Could you check a few things on this drawing? It's one solid part, dimensions in mm from its lowest x, y, z. A direction names the side the tool comes from. Give positions to 0.01 mm unless a question says otherwise; leave off trailing zeros. Loops run counter-clockwise (first coordinate to the right, second up) from the corner with the lowest first, then second, coordinate; pieces in that order, holes last.
1. Imagine slicing it at D-D (z = 23). List the corners of the cut face in (x, y) for me.
2. For the marked faces 1 and 2, which set-ups out of +Z, -Z, +X, -X, +Y, -Y let a thin tool reach every point of the face, with its end or its side?
3. For P1, Ø2.5, axis at y = 6.35, z = 19.05, coming from the -X side; P2, Ø1, axis at x = 1, y = 4.5, coming from the +Z side (3 decimals), each with a flat end and sliding along its axis, tell me the tip position at first contact or that it passes through.
4. Imagine slicing it at A-A (z = 5.25). List the corners of the cut face in (x, y) for me.
5. I need wall thicknesses on line 1 along Y through (x, z) = (1, 19.05); line 2 along Y through (x, z) = (1.9, 2.5); line 3 along Z through (x, y) = (2.8, 4.25). Which ranges of each line are inside material? Lowest first, please.
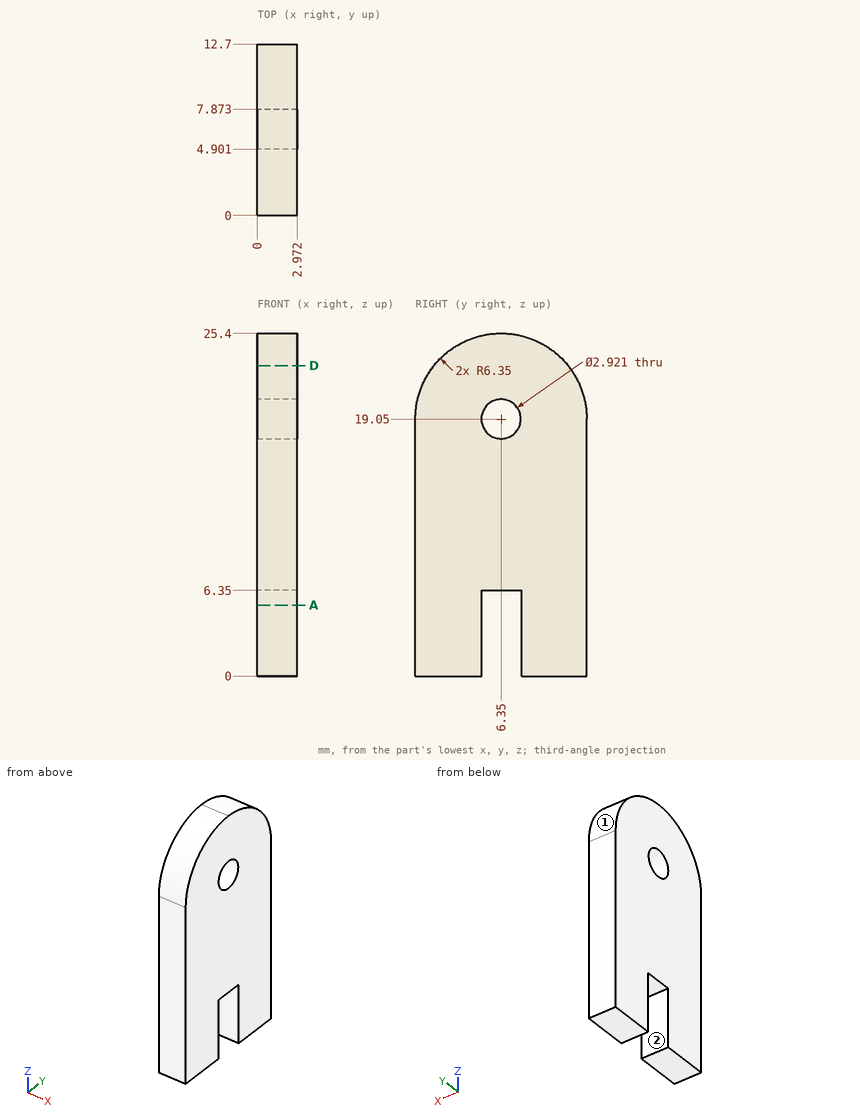
Derived:
1. outline: (0, 1.38) - (2.97, 1.38) - (2.97, 11.32) - (0, 11.32) - close
2. face 1: +Z, +X, -X, +Y
2. face 2: -Z, +X, -X
3. P1: passes through
3. P2: stops at z = 25.255
4. outline: (0, 0) - (2.97, 0) - (2.97, 4.9) - (0, 4.9) - close; (0, 7.87) - (2.97, 7.87) - (2.97, 12.7) - (0, 12.7) - close
5. line 1: y = 0 to 4.89, 7.81 to 12.7
5. line 2: y = 0 to 4.9, 7.87 to 12.7
5. line 3: z = 0 to 25.04
